The model under review builds one solid part; all positions refer to its coordinate system, in mm. A direction names the side the tool comes from. Give positions to 0.01 mm unless a question says otherwise; leave off trailing zeros. Write each loop counter-clockwise with the first axis right and the second up, starting at its lowest first coordinate (ties: lowest second). Pieces come first, ordered by that corner, then holes. Notation, with made-up numbers: M 67,27 L 88,27 A26 ccw 88,65 Z; hole C 51,-8 d1. An arc over 180 degrees is marked long. Write item = value, one per line. Start each with the question number.
```python
from build123d import *

# Parameters (mm, degrees)
EXTRUDE_THIN1_DEPTH = 571.5
FILLET1_R           = 1.27


with BuildPart() as part:
    # Sketch1 → Extrude-Thin1 (new body)
    with BuildSketch(Plane.XY):
        with BuildLine():
            Line((0, 6.35), (0, 0))
            Line((0, 0), (-6.35, 0))
            Line((-6.35, 0), (-6.35, 28.575))
            Line((-6.35, 28.575), (-9.525, 28.575))
            ThreePointArc((-9.525, 28.575), (-13.244743879, 37.555256121), (-22.225, 41.275))
            Line((-22.225, 41.275), (-22.225, 57.15))
            Line((-22.225, 57.15), (0, 57.15))
            Line((0, 57.15), (0, 50.8))
            Line((0, 50.8), (-1.27, 50.8))
            Line((-1.27, 50.8), (-1.27, 55.88))
            Line((-1.27, 55.88), (-20.955, 55.88))
            Line((-20.955, 55.88), (-20.955, 42.487152961))
            ThreePointArc((-20.955, 42.487152961), (-12.346718267, 38.453281733), (-8.312847039, 29.845))
            Line((-8.312847039, 29.845), (-5.08, 29.845))
            Line((-5.08, 29.845), (-5.08, 1.27))
            Line((-5.08, 1.27), (-1.27, 1.27))
            Line((-1.27, 1.27), (-1.27, 6.35))
            Line((-1.27, 6.35), (0, 6.35))
        make_face()
    extrude(amount=-EXTRUDE_THIN1_DEPTH)

    # Fillet1
    fillet1_edges = [part.edges().sort_by_distance(p)[0] for p in [
        (-5.08, 29.845, -285.75),
        (0, 0, -285.75),
        (-6.35, 0, -285.75),
        (-9.525, 28.575, -285.75),
        (-22.225, 41.275, -285.75),
        (-22.225, 57.15, -285.75),
        (0, 57.15, -285.75),
    ]]
    fillet(fillet1_edges, radius=FILLET1_R)


solid = part.part
```
Item 1: For faces 1 (the cylindrical face through (-12.443, 38.549, -281.75)), 2 (the flat face through (-9.4, 32.9, -571.5)), 3 (the flat face through (-5.08, 15, -282)), 4 (the flat face through (-6.35, 15, -282)), list the 3-axis set-ups (+Z, -Z, +X, -X, +Y, -Y) from which the entire face can be reached by the end or side of a thin tool; tool diameter is ignored.
Item 2: The part is to be moulded in two halves that separate along X. For faces 5 (the flat face through (-22.225, 49, -282)), 6 (the flat face through (-9.4, 32.9, 0)), 7 (the flat face through (-11, 55.88, -282)), say which applies: released by +X, released by -X, zero draft, split by the parting line, or undercut.
Item 3: We need section A-A, the plane x = -13.5. Write out the cut boundary in (y, z), and give its area (3 significant figures).
Item 4: We need section B-B, the plane z = -73.5. Write out the cut boundary in (x, y) (3 decimals).
Item 5: Clearance check with flat-ended pins moving along their axes: P1, Ø6, axis at x = -11.5, z = -306, coming from the -Y side; P2, Ø1.5, axis at x = -7.5, y = 21, coming from the -Z side; P3, Ø0.6, axis at x = -0.5, z = -163, coming from the -Y side; P4, Ø1, axis at x = -0.5, z = -340, coming from the +Y side. State where each tip first meets the part, or that it passes through.
Item 6: To check wall thickness, follow probe 1 along Y at (x, z) = (-4.5, -346.5); probe 2 along X at (y, z) = (5, -265); probe 3 along Y at (x, z) = (-7.25, -124) (3 decimals). State the ranges of each line that lie inside material, in increasing order. Write a range as [from, to].
Item 7: We need section C-C, the plane y = 23.5. Write out the cut boundary in (x, z).
Worked out:
q1.face_1 = +Z, -Z, +X
q1.face_2 = -Z, +X, -X, +Y, -Y
q1.face_3 = +Z, -Z
q1.face_4 = +Z, -Z, -X, -Y
q2.face_5 = released by -X
q2.face_6 = zero draft
q2.face_7 = undercut
q3.outline = M 37.8,-571.5 L 39.49,-571.5 L 39.49,0 L 37.8,0 Z; M 55.88,-571.5 L 57.15,-571.5 L 57.15,0 L 55.88,0 Z
q3.area = 1,690 mm²
q4.outline = M -22.225,42.487 A1.27 ccw -21.07,41.222 A12.7 cw -9.578,29.73 A1.27 ccw -8.313,28.575 L -6.35,28.575 L -6.35,1.27 A1.27 ccw -5.08,0 L -1.27,0 A1.27 ccw 0,1.27 L 0,6.35 L -1.27,6.35 L -1.27,1.27 L -5.08,1.27 L -5.08,28.575 A1.27 ccw -6.35,29.845 L -8.313,29.845 A13.97 ccw -20.955,42.487 L -20.955,55.88 L -1.27,55.88 L -1.27,50.8 L 0,50.8 L 0,55.88 A1.27 ccw -1.27,57.15 L -20.955,57.15 A1.27 ccw -22.225,55.88 Z
q5.P1 = 28.59
q5.P2 = through
q5.P3 = 0.09
q5.P4 = 57.12
q6.probe_1 = [0, 1.27], [55.88, 57.15]
q6.probe_2 = [-6.35, -5.08], [-1.27, 0]
q6.probe_3 = [28.575, 29.845], [55.88, 57.15]
q7.outline = M -6.35,-571.5 L -5.08,-571.5 L -5.08,0 L -6.35,0 Z
